```python
from build123d import *

# Parameters (mm, degrees)
SKETCH_1_W          = 250
SKETCH_1_H          = 380
SKETCH_1_R          = 9
SKETCH_1_R_2        = 2
SKETCH_1_R_3        = 1.5
SKETCH_1_R_4        = 3
EXTRUDE_3_DEPTH     = 25
CUT_EXTRUDE_1_DEPTH = 416
SKETCH_3_4_R        = 4
CUT_EXTRUDE_2_DEPTH = 55
SKETCH_5_W          = 76.418543054
SKETCH_5_H          = 18.162254628
EXTRUDE_4_DEPTH     = 12
SKETCH_6_W          = 9.937837438
SKETCH_6_H          = 197.728696601
EXTRUDE_5_DEPTH     = 12
SKETCH_7_W          = 21.060874429
SKETCH_7_H          = 111.734651623
EXTRUDE_6_DEPTH     = 12
SKETCH_8_W          = 15.76346628
SKETCH_8_H          = 76.418543054
EXTRUDE_7_DEPTH     = 5
SKETCH_9_W          = 10.965889587
SKETCH_9_H          = 75.390490905
EXTRUDE_8_DEPTH     = 5
SKETCH_10_W         = 21.30480461
SKETCH_10_H         = 26.996927979
SKETCH_10_R         = 6
EXTRUDE_11_DEPTH    = 11
FILLET_1_R          = 4


with BuildPart() as part:
    # 草图1 → 凸台-拉伸3 (new body)
    with BuildSketch(Plane.XY):
        with Locations((125.613842041, 190.076299127)):
            Rectangle(SKETCH_1_W, SKETCH_1_H)
        with Locations((13, 12.5)):
            Circle(SKETCH_1_R, mode=Mode.SUBTRACT)
        with Locations((237, 12.5)):
            Circle(SKETCH_1_R, mode=Mode.SUBTRACT)
        with Locations((5, 360)):
            Circle(SKETCH_1_R_2, mode=Mode.SUBTRACT)
        with Locations((5, 260)):
            Circle(SKETCH_1_R_2, mode=Mode.SUBTRACT)
        with Locations((15, 360)):
            Circle(SKETCH_1_R_2, mode=Mode.SUBTRACT)
        with Locations((15, 260)):
            Circle(SKETCH_1_R_2, mode=Mode.SUBTRACT)
        with Locations((89, 280)):
            Circle(SKETCH_1_R_3, mode=Mode.SUBTRACT)
        with Locations((113, 280)):
            Circle(SKETCH_1_R_3, mode=Mode.SUBTRACT)
        with Locations((137, 280)):
            Circle(SKETCH_1_R_3, mode=Mode.SUBTRACT)
        with Locations((161, 280)):
            Circle(SKETCH_1_R_3, mode=Mode.SUBTRACT)
        with Locations((45, 110)):
            Circle(SKETCH_1_R_4, mode=Mode.SUBTRACT)
        with Locations((45, 170)):
            Circle(SKETCH_1_R_4, mode=Mode.SUBTRACT)
        with Locations((205, 170)):
            Circle(SKETCH_1_R_4, mode=Mode.SUBTRACT)
        with Locations((205, 110)):
            Circle(SKETCH_1_R_4, mode=Mode.SUBTRACT)
        with Locations((245, 345)):
            Circle(SKETCH_1_R_3, mode=Mode.SUBTRACT)
        with Locations((245, 285)):
            Circle(SKETCH_1_R_3, mode=Mode.SUBTRACT)
        with Locations((245, 225)):
            Circle(SKETCH_1_R_3, mode=Mode.SUBTRACT)
        with Locations((245, 165)):
            Circle(SKETCH_1_R_3, mode=Mode.SUBTRACT)
    extrude(amount=EXTRUDE_3_DEPTH)

    # 草图3 → 切除-拉伸1 (cut)
    with BuildSketch(Plane(origin=(0, 380.076299127, 0), x_dir=(1, 0, 0), z_dir=(0, 1, 0))):
        Polygon((71.5, -9), (71.5, 0), (58.5, 0), (58.5, -9), (55, -9), (55, -18), (75, -18), (75, -9), align=None)
        Polygon((191.5, 0), (178.5, 0), (178.5, -9), (175, -9), (175, -18), (195, -18), (195, -9), (191.5, -9), align=None)
    extrude(amount=-CUT_EXTRUDE_1_DEPTH, mode=Mode.SUBTRACT)

    # 草图3<4> → 切除-拉伸2 (cut)
    with BuildSketch(Plane(origin=(0, 380.076299127, 0), x_dir=(1, 0, 0), z_dir=(0, 1, 0))):
        with Locations(Location((95, -12.5, 0), (0, 0, 270))):
            Circle(SKETCH_3_4_R)
        with Locations(Location((155, -12.5, 0), (0, 0, 270))):
            Circle(SKETCH_3_4_R)
        with Locations(Location((225, -12.5, 0), (0, 0, 270))):
            Circle(SKETCH_3_4_R)
        with Locations(Location((25, -12.5, 0), (0, 0, 270))):
            Circle(SKETCH_3_4_R)
    extrude(amount=-CUT_EXTRUDE_2_DEPTH, mode=Mode.SUBTRACT)

    # 草图5 → 凸台-拉伸4 (add)
    with BuildSketch(Plane(origin=(0, 0, 0), x_dir=(-1, 0, 0), z_dir=(0, 0, -1))):
        with Locations((-124.414447867, 279.859520114)):
            Rectangle(SKETCH_5_W, SKETCH_5_H)
    extrude(amount=-EXTRUDE_4_DEPTH)

    # 草图6 → 凸台-拉伸5 (add)
    with BuildSketch(Plane(origin=(0, 0, 0), x_dir=(-1, 0, 0), z_dir=(0, 0, -1))):
        with Locations((-244.34867248, 253.130164248)):
            Rectangle(SKETCH_6_W, SKETCH_6_H)
    extrude(amount=-EXTRUDE_5_DEPTH)

    # 草图7 → 凸台-拉伸6 (add)
    with BuildSketch(Plane(origin=(0, 0, 0), x_dir=(-1, 0, 0), z_dir=(0, 0, -1))):
        with Locations((-11.144279256, 310.45109449)):
            Rectangle(SKETCH_7_W, SKETCH_7_H)
    extrude(amount=-EXTRUDE_6_DEPTH)

    # 草图8 → 凸台-拉伸7 (add)
    with BuildSketch(Plane(origin=(0, 0, 0), x_dir=(-1, 0, 0), z_dir=(0, 0, -1))):
        with Locations((-204.431173441, 138.673691692)):
            Rectangle(SKETCH_8_W, SKETCH_8_H)
    extrude(amount=-EXTRUDE_7_DEPTH)

    # 草图9 → 凸台-拉伸8 (add)
    with BuildSketch(Plane(origin=(0, 0, 0), x_dir=(-1, 0, 0), z_dir=(0, 0, -1))):
        with Locations((-45.425774442, 139.530401815)):
            Rectangle(SKETCH_9_W, SKETCH_9_H)
    extrude(amount=-EXTRUDE_8_DEPTH)

    # 草图10 → 凸台-拉伸11 (add)
    # profile 1 of 2: a face of its own
    with BuildSketch(Plane(origin=(0, 0, 0), x_dir=(-1, 0, 0), z_dir=(0, 0, -1))):
        with Locations((-236.946967286, 15.123600302)):
            Rectangle(SKETCH_10_W, SKETCH_10_H)
        with Locations((-237, 12.5)):
            Circle(SKETCH_10_R, mode=Mode.SUBTRACT)
    # profile 2 of 2: a face of its own
    with BuildSketch(Plane(origin=(0, 0, 0), x_dir=(-1, 0, 0), z_dir=(0, 0, -1))):
        with Locations((-13.053032714, 15.123600302)):
            Rectangle(SKETCH_10_W, SKETCH_10_H)
        with Locations((-13, 12.5)):
            Circle(SKETCH_10_R, mode=Mode.SUBTRACT)
    extrude(amount=-EXTRUDE_11_DEPTH)

    # 圆角1
    # the kernel refuses this fillet: 4 mm, written as the material it takes off along each edge
    with BuildSketch(Plane(origin=(-9.386157959, 0.076299127, 25), x_dir=(0, 0, -1), z_dir=(1, 0, 0))) as fillet_1_piece_1:
        with BuildLine():
            CenterArc((FILLET_1_R, FILLET_1_R), FILLET_1_R, 180, 90)
            Line((0, FILLET_1_R), (0, 0))
            Line((0, 0), (FILLET_1_R, 0))
        make_face()
    extrude(amount=270, mode=Mode.SUBTRACT)


solid = part.part
```
CAD build for the part. Positions are in the model's coordinates, mm. A direction names the side the tool comes from. Round coordinates to 2 decimals unless told otherwise and drop trailing zeros. Loops run counter-clockwise (first coordinate to the right, second up) from the corner with the lowest first, then second, coordinate; pieces in that order, holes last. Notation, with made-up numbers: M -20.75,58.5 L 24.25,58.5 A17 ccw 24.25,62.5 Z; hole C -24,57.25 d8. An arc over 180 degrees is marked long. Return JSON: item names as keys, results as strings. Group by question number.
(1) Drop flat-ended pins along their axis: P1, Ø2, axis at x = 4.5, y = 359.5, coming from the +Z side; P2, Ø3.5, axis at x = 45, y = 170, coming from the -Z side; P3, Ø5.5, axis at x = 205, y = 110, coming from the +Z side. Give the stop position or say it passes through.
(2) Saw through at A-A, the plane y = 12.5. Give the number of separate pieces and of enclosed holes in the cut face, and give its area (3 significant figures).
(3) Tool access for faces 3 (the flat face through (191.5, 193, 5)), 4 (the flat face through (195, 193, 14)), 5 (the cylindrical face through (158.966, 352.961, 11.979)): list every direction of +Z, -Z, +X, -X, +Y, -Y with a clear straight run to the whole face (end or side of a thin tool).
(4) Saw through at B-B, the plane y = 76. List the corners of the cut face in (x, z).
(5) Mould opens along X. For faces 1 (the cylindrical face through (91.095, 352.961, 11.633)), 2 (the flat face through (221, 193, 0)) say: +X half, -X half, draft (parallel to the pull), parting line (faces both ways), or undercut.
(6) Wall check: probe 1 along X at (y, z) = (51.5, 2.5); probe 2 along X at (y, z) = (278, 11.5); probe 3 along X at (y, z) = (165, 15.5). Give the ranges that are in metal, low to high. Write a range as [from, to].
Answer list:
{
 "1": {"P1": "z = 12", "P2": "z = 0", "P3": "z = 5"},
 "2": {"separate pieces": "3", "enclosed holes": "0", "area": "4,890 mm2"},
 "3": {"face 3": "-Z, +Y, -Y", "face 4": "+Y, -Y", "face 5": "+Y"},
 "4": {"outline": "M 0.61,0 L 58.5,0 L 58.5,9 L 55,9 L 55,18 L 75,18 L 75,9 L 71.5,9 L 71.5,0 L 178.5,0 L 178.5,9 L 175,9 L 175,18 L 195,18 L 195,9 L 191.5,9 L 191.5,0 L 250.61,0 L 250.61,25 L 0.61,25 Z"},
 "5": {"face 1": "undercut", "face 2": "draft"},
 "6": {"probe 1": "[0.61, 58.5], [71.5, 178.5], [191.5, 250.61]", "probe 2": "[0.61, 55], [75, 175], [195, 250.61]", "probe 3": "[0.61, 55], [75, 175], [195, 243.5], [246.5, 250.61]"}
}
